Autodesk Inventor part; units mm, degrees
ref_plane "Work Plane1" through (0, 0, 5) normal (0, 0, 1) x (1, 0, 0)
ref_plane "YZ Plane" through (0, 0, 0) normal (1, 0, 0) x (0, 1, 0)
ref_plane "XZ Plane" through (0, 0, 0) normal (0, 1, 0) x (-1, 0, 0)
sketch "Sketch1" plane through (0, 0, 0) normal (0, 1, 0) x (-1, 0, 0)
  circle A0 centre (0, 0) radius 3.175
  arc A1 (4.1151, 2.84) -> (3.5707, 3.5) centre (0, 0) ccw
  arc A2 (-11, 3.5) -> (-11, -3.5) centre (-11, 0) ccw
  line L0 (0, 0) -> (0, -5) construction
  arc A3 (4.1151, -2.84) -> (4.1151, 2.84) centre (0, 0) ccw
  line L1 (-7, 0) -> (-11, 0) construction
  line L2 (-7, -1.5) -> (-11, -1.5)
  line L3 (-11, 1.5) -> (-7, 1.5)
  arc A4 (-7, -1.5) -> (-7, 1.5) centre (-7, 0) ccw
  arc A5 (-11, 1.5) -> (-11, -1.5) centre (-11, 0) ccw
  line L4 (-11, 3.5) -> (-3.5707, 3.5)
  line L5 (-11, -3.5) -> (-3.5707, -3.5)
  line L6 (0, 0) -> (0, 3.175) construction
  arc A6 (11, -3.5) -> (11, 3.5) centre (11, 0) ccw
  line L7 (7, -1.5) -> (11, -1.5)
  line L8 (11, 1.5) -> (7, 1.5)
  arc A7 (7, 1.5) -> (7, -1.5) centre (7, 0) ccw
  arc A8 (11, -1.5) -> (11, 1.5) centre (11, 0) ccw
  line L9 (11, 3.5) -> (3.5707, 3.5)
  line L10 (11, -3.5) -> (3.5707, -3.5)
  arc A9 (3.5707, 3.5) -> (3.5707, -3.5) centre (0, 0) ccw
  arc A10 (3.5707, -3.5) -> (4.1151, -2.84) centre (0, 0) ccw
  point P0 (-9, 0)
  dimension "d0" = 6.35
  dimension "d1" = 10
  dimension "d6" = 3.5
  dimension "d15" = 3
  dimension "d16" = 4
  dimension "d17" = 7
extrude "Extrusion1" add sketch "Sketch1" against normal blind 2
extrude "Extrusion2" add sketch "Sketch1" along normal blind 6 contours A3 A10 A9 A1
sketch "Sketch2" plane through (0, 0, 0) normal (0, 0, 1) x (1, 0, 0)
  circle A0 centre (0, 3) radius 1.5
  line L0 (5, 6) -> (5, 0)
  point P0 (0, 0)
  point P1 (5, 3)
  dimension "d11" = 3
extrude "Extrusion3" cut sketch "Sketch2" along normal through all both and the other way through all
ref_plane "Work Plane1" through (0, 0, 5) normal (0, 0, 1) x (1, 0, 0)
properties part number "EncoderWheelAdapterSlotted" material "ABS Plastic"
Geometry: final body of the model. Coordinates: model frame, mm. A direction names the side the tool comes from. Coordinates: 2 decimals unless noted, no trailing zeros. Order: outer loops, then holes, each group sorted by start corner. A loop starts at its lowest first (then second) coordinate and runs counter-clockwise, first axis right, second up. Notation, with made-up numbers: (-20.5, -7.5) -> (-4.5, -7.5) arc R21 cw to (-4.5, 22.5) -> close; hole circle Ø7 at (31, 23.25). An arc over 180 degrees is marked (long way). Use CSV: the item, a comma, the result in double quotes.
1) Section B-B on x = -12. Output: boundary loops of the cut face in (y, z).
Findings:
outline,"(-2, -3.35) -> (0, -3.35) -> (0, -1.12) -> (-2, -1.12) -> close; (-2, 1.12) -> (0, 1.12) -> (0, 3.35) -> (-2, 3.35) -> close"
2) Section D-D on x = -0.5. Output: boundary loops of the cut face in (y, z).
Findings:
outline,"(-2, -4.97) -> (1.59, -4.97) -> (1.59, -3.14) -> (-2, -3.14) -> close; (-2, 3.14) -> (1.59, 3.14) -> (1.59, 4.97) -> (-2, 4.97) -> close; (4.41, -4.97) -> (6, -4.97) -> (6, -3.14) -> (4.41, -3.14) -> close; (4.41, 3.14) -> (6, 3.14) -> (6, 4.97) -> (4.41, 4.97) -> close"
3) Section C-C on y = -0.5. Output: boundary loops of the cut face in (x, z) (3 decimals), then the cut area to 3 significant figures.
Findings:
outline,"(-11, -3.5) -> (-3.571, -3.5) arc R5 ccw to (3.571, -3.5) -> (11, -3.5) arc R3.5 ccw to (11, 3.5) -> (3.571, 3.5) arc R5 ccw to (-3.571, 3.5) -> (-11, 3.5) arc R3.5 ccw to start; hole (-11, -1.5) -> (-7, -1.5) arc R1.5 ccw to (-7, 1.5) -> (-11, 1.5) arc R1.5 ccw to start; hole circle Ø6.35 at (0, 0); hole (7, -1.5) -> (11, -1.5) arc R1.5 ccw to (11, 1.5) -> (7, 1.5) arc R1.5 ccw to start"
area,"137 mm^2"
4) Line query: line 1 (Y direction, x = 0, z = -4.3); line 2 (Z direction, x = 0, y = 0.5) (3 decimals). Output: solid intervals per line, ascending.
Findings:
line 1,"y = -2 to 1.5, 4.5 to 6"
line 2,"z = -5 to -3.175, 3.175 to 5"
5) Access query for faces 4 (the flat face through (7, -1, 3.5)), 5 (the cylindrical face through (1.43, 3.45, -3.88)), 6 (the flat face through (3.4, -2, 0.1)), 7 (the flat face through (9, -1, -1.5)), 8 (the cylindrical face through (5, 2, 0)). Directions: +Z, -Z, +X, -X, +Y, -Y. A direction counts if a zero-diameter tool reaches every point of the face in a straight line with its end or side. Return the directions, or none.
Findings:
face 4,"+Z, +X, +Y, -Y"
face 5,"+Z, -Z"
face 6,"+Z, -Z, +X, -X, -Y"
face 7,"+Y, -Y"
face 8,"+Y"
6) Mould query, pull axis Z, two halves, no side actions, for faces 1 (the cylindrical face through (-5, 3, 0)), 2 (the cylindrical face through (-1.707, 1.944, -2.677)), 3 (the flat face through (9, 0, 2)). Classes: +Z half, -Z half, draft (parallel to the pull), parting line (faces both ways), or undercut.
Findings:
face 1,"parting line"
face 2,"undercut"
face 3,"draft"
7) Section A-A on z = 0. Output: boundary loops of the cut face in (x, y) (3 decimals).
Findings:
outline,"(-14.5, -2) -> (-12.5, -2) -> (-12.5, 0) -> (-14.5, 0) -> close; (-5.5, -2) -> (-3.175, -2) -> (-3.175, 6) -> (-5, 6) -> (-5, 0) -> (-5.5, 0) -> close; (3.175, -2) -> (5.5, -2) -> (5.5, 0) -> (5, 0) -> (5, 6) -> (3.175, 6) -> close; (12.5, -2) -> (14.5, -2) -> (14.5, 0) -> (12.5, 0) -> close"
8) Pin query (flat end, axial travel): pin 1 Ø4 at (x, y) = (0, 3) entering from +Z; pin 2 Ø4 at (x, y) = (8.5, 1.5) entering from -Z; pin 3 Ø2 at (x, y) = (-6, -0.5) entering from +Z; pin 4 Ø1 at (x, z) = (9.5, 1.5) entering from +Y. Return the tip coordinate at first contact, or that it passes through.
Findings:
pin 1,"stops at z = 5"
pin 2,"stops at z = -3.5"
pin 3,"stops at z = 3.5"
pin 4,"stops at y = 0"
